```python
from build123d import *

# Parameters (mm, degrees)
SKETCH1_R           = 3.5
BOSS_EXTRUDE1_DEPTH = 4
CUT_EXTRUDE1_DEPTH  = 2
SKETCH3_R           = 2
BOSS_EXTRUDE2_DEPTH = 25


with BuildPart() as part:
    # Sketch1 → Boss-Extrude1 (new body)
    with BuildSketch(Plane.XY):
        Circle(SKETCH1_R)
    extrude(amount=BOSS_EXTRUDE1_DEPTH)

    # Sketch2 → Cut-Extrude1 (cut)
    with BuildSketch(Plane.XY.offset(4)):
        Polygon((0, -1.732050808), (1.5, -0.866025404), (1.5, 0.866025404), (0, 1.732050808), (-1.5, 0.866025404), (-1.5, -0.866025404), align=None)
    extrude(amount=-CUT_EXTRUDE1_DEPTH, mode=Mode.SUBTRACT)

    # Sketch3 → Boss-Extrude2 (add)
    with BuildSketch(Plane(origin=(0, 0, 0), x_dir=(-1, 0, 0), z_dir=(0, 0, -1))):
        Circle(SKETCH3_R)
    extrude(amount=BOSS_EXTRUDE2_DEPTH)


solid = part.part
```
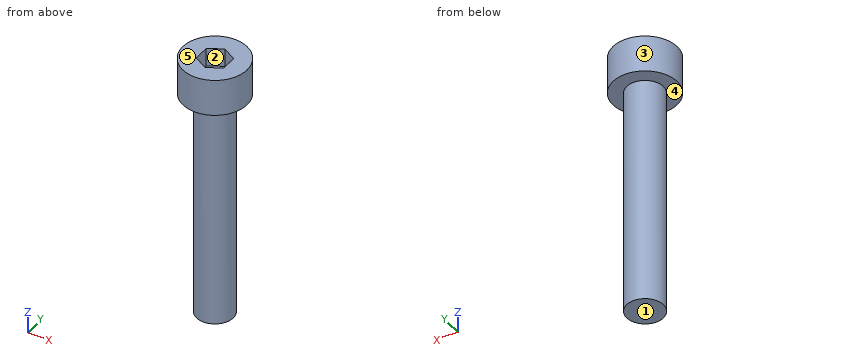
Here's how the part is built. I have some questions about the finished solid (model axes, mm). Face numbers are marked on the shaded views. A direction names the side the tool comes from. Coordinates: 2 decimals unless noted, no trailing zeros. Write each loop counter-clockwise with the first axis right and the second up, starting at its lowest first coordinate (ties: lowest second). Pieces come first, ordered by that corner, then holes. Notation, with made-up numbers: (-2.75, -35) - (17.25, -35) arc R14 cw to (17.25, -11) - close; hole circle Ø2 at (72, 51.25). An arc over 180 degrees is marked (long way). One line per item, written item: value.
1) Suppose I cut it at D-D on z = -13.5. Write out the boundary of the cut face in (x, y), and give its area (3 significant figures).
Model answer:
outline: circle Ø4 at (0, 0)
area: 12.6 mm²
2) Suppose I cut it at B-B on x = -1. Write out the boundary of the cut face in (y, z), and give its area (3 significant figures).
Model answer:
outline: (-3.35, 0) - (-1.73, 0) - (-1.73, -25) - (1.73, -25) - (1.73, 0) - (3.35, 0) - (3.35, 4) - (1.15, 4) - (1.15, 2) - (-1.15, 2) - (-1.15, 4) - (-3.35, 4) - close
area: 109 mm²
3) On a 3-axis mill with a long thin cutter (end or side, diameter ignored), from which of +Z, -Z, +X, -X, +Y, -Y can I reach the whole of each face in a straight line? I mean the marked faces 4 and 5. Say none if no direction works.
Model answer:
face 4: -Z
face 5: +Z, +X, -X, +Y, -Y
4) I need wall thicknesses on line 1 along Y through (x, z) = (-1, -9); line 2 along Z through (x, y) = (2, 1.5); line 3 along Z through (x, y) = (-1, 1). Which ranges of each line are inside material? Lowest first, please.
Model answer:
line 1: y = -1.73 to 1.73
line 2: z = 0 to 4
line 3: z = -25 to 2
5) We'd pull the mould along X, two halves only. Please class the marked faces 1, 2 and 3: pulls with the +X half, pulls with the -X half, needs draft (parallel to the pull), parting line crosses it, or undercut.
Model answer:
face 1: needs draft
face 2: undercut
face 3: parting line crosses it
6) Suppose I cut it at C-C on z = 0.75. Write out the boundary of the cut face in (x, y), and give its area (3 significant figures).
Model answer:
outline: circle Ø7 at (0, 0)
area: 38.5 mm²
7) Suppose I cut it at A-A on y = 0. Write out the boundary of the cut face in (x, z), and give its area (3 significant figures).
Model answer:
outline: (-3.5, 0) - (-2, 0) - (-2, -25) - (2, -25) - (2, 0) - (3.5, 0) - (3.5, 4) - (1.5, 4) - (1.5, 2) - (-1.5, 2) - (-1.5, 4) - (-3.5, 4) - close
area: 122 mm²
8) I'm going to push flat-ended pins straight in: P1, Ø2, axis at y = 2.5, z = -5, coming from the +X side; P2, Ø0.9, axis at x = 0.5, y = 0, coming from the +Z side; P3, Ø4, axis at y = 1.5, z = -6.5, coming from the -X side. Where does each tip first touch, or does it pass through?
Model answer:
P1: stops at x = 1.32
P2: stops at z = 2
P3: stops at x = -2
